Can you work these out from the drawing? Everything is in mm from the part's minimum corner. A direction names the side the tool comes from. Round coordinates to 2 decimals unless told otherwise and drop trailing zeros. Write each loop counter-clockwise with the first axis right and the second up, starting at its lowest first coordinate (ties: lowest second). Pieces come first, ordered by that corner, then holes. Notation, with made-up numbers: (6, -36) -> (31, -36) arc R21 cw to (31, -28) -> close; hole circle Ø4 at (75, 50). An arc over 180 degrees is marked (long way). Answer as CSV lines item,"result".
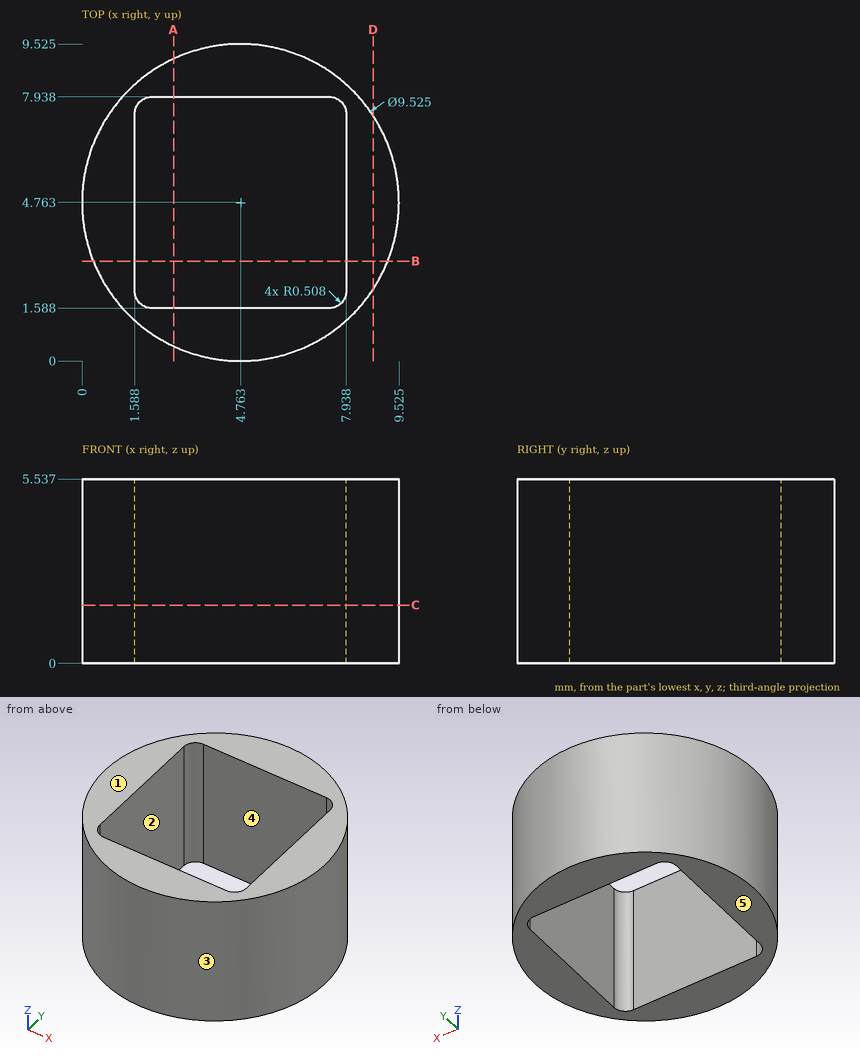
Item 1: Suppose I cut it at C-C, the plane z = 1.75. List the corners of the cut face in (x, y) for me (1 decimal).
Results found:
outline,"circle Ø9.5 at (4.8, 4.8); hole (1.6, 2.1) arc R0.5 ccw to (2.1, 1.6) -> (7.4, 1.6) arc R0.5 ccw to (7.9, 2.1) -> (7.9, 7.4) arc R0.5 ccw to (7.4, 7.9) -> (2.1, 7.9) arc R0.5 ccw to (1.6, 7.4) -> close"
Item 2: Suppose I cut it at B-B, the plane y = 3. List the corners of the cut face in (x, z) for me.
Results found:
outline,"(0.34, 0) -> (1.59, 0) -> (1.59, 5.54) -> (0.34, 5.54) -> close; (7.94, 0) -> (9.19, 0) -> (9.19, 5.54) -> (7.94, 5.54) -> close"
Item 3: Suppose I cut it at A-A, the plane x = 2.75. List the corners of the cut face in (y, z) for me.
Results found:
outline,"(0.45, 0) -> (1.59, 0) -> (1.59, 5.54) -> (0.45, 5.54) -> close; (7.94, 0) -> (9.08, 0) -> (9.08, 5.54) -> (7.94, 5.54) -> close"
Item 4: Suppose I cut it at D-D, the plane x = 8.75. List the corners of the cut face in (y, z) for me.
Results found:
outline,"(2.16, 0) -> (7.37, 0) -> (7.37, 5.54) -> (2.16, 5.54) -> close"
Item 5: For the marked faces 4 and 5, which set-ups out of +Z, -Z, +X, -X, +Y, -Y let a thin tool reach every point of the face, with its end or its side?
Results found:
face 4,"+Z, -Z"
face 5,"-Z, +X, -X, +Y, -Y"
Item 6: If we mould it in two halves opening along X, with no side actions, what happens to the marked faces 1, 2 and 3? For each: pulls with the +X half, pulls with the -X half, needs draft (parallel to the pull), parting line crosses it, or undercut.
Results found:
face 1,"needs draft"
face 2,"undercut"
face 3,"parting line crosses it"
Item 7: Will these pins go through, and if not, where does the flat tip stop? pin 1 (2 mm diameter, centred on x = 4.5, y = 5.5, fed in from +Z); pin 2 (1.5 mm diameter, centred on y = 8, z = 1, fed in from +X) (1 decimal); pin 3 (1.5 mm diameter, centred on x = 1.5, z = 1.5, fed in from -Y).
Results found:
pin 1,"passes through"
pin 2,"stops at x = 8.8"
pin 3,"stops at y = 0.72"
Item 8: I need wall thicknesses on L1, parallel to Y at x = 7.5, z = 1.1 (1 decimal); L2, parallel to Y at x = 7, z = 4.5 (1 decimal); L3, parallel to X at y = 6.5, z = 3 (1 decimal). Which ranges of each line are inside material? Lowest first, please.
Results found:
L1,"y = 0.9 to 1.6, 7.9 to 8.7"
L2,"y = 0.6 to 1.6, 7.9 to 9"
L3,"x = 0.3 to 1.6, 7.9 to 9.2"
